Part model, mm, in its own coordinate system. Face numbers are marked on the shaded views. A direction names the side the tool comes from. Round coordinates to 2 decimals unless told otherwise and drop trailing zeros. Loops run counter-clockwise (first coordinate to the right, second up) from the corner with the lowest first, then second, coordinate; pieces in that order, holes last.
1) Drop flat-ended pins along their axis: P1, Ø3, axis at y = 2.5, z = -12, coming from the +X side; P2, Ø6, axis at x = -5.5, z = -9, coming from the -Y side; P3, Ø4, axis at x = -2, y = 13, coming from the -Z side. Give the stop position or say it passes through.
2) 3-axis set-ups, long thin cutter, end or side, ignore diameter. For the marked faces 4, 5 and 6: which of +Z, -Z, +X, -X, +Y, -Y reach the whole face in a straight line?
3) Band-saw the part on B-B, the plane z = 0. Write the cut outline in (x, y), then the cut area to 3 significant figures.
4) Mould opens along X. For the marked faces 1, 2 and 3 say: +X half, -X half, draft (parallel to the pull), parting line (faces both ways), or undercut.
5) Band-saw the part on C-C, the plane y = 7.75. Write the cut outline in (x, z), then the cut area to 3 significant figures.
6) Probe line 1 (Y direction, x = 0, z = 9.5); line 2 (X direction, y = 6.25, z = 0); line 3 (X direction, y = 0.5, z = 0). List the from-to ranges inside material, lowest first.
7) Band-saw the part on D-D, the plane y = 4. Write the cut outline in (x, z).
8) Band-saw the part on A-A, the plane x = 0. Write the cut outline in (y, z), then the cut area to 3 significant figures.
from build123d import *

# Parameters (mm, degrees)
SKETCH1_R             = 7.5
BASE_CYLINDER_DEPTH   = 15.4
LED_HOLDER_DEPTH      = 7.5
LED_HOLDER_DEPTH_BACK = 22.5
F_3DSKETCH2_R         = 3.5
SKETCH2_R             = 6.05
CUT_EXTRUDE1_DEPTH    = 14.2
CUT_EXTRUDE2_REACH    = 24.769
SKETCH3_R             = 1.75
SKETCH4_R             = 2.5
CUT_EXTRUDE3_DEPTH    = 35.545766898


with BuildPart() as part:
    # Sketch1 → base-cylinder (new body)
    with BuildSketch(Plane(origin=(0, 0, 0), x_dir=(1, 0, 0), z_dir=(0, 1, 0))):
        with Locations(Location((0, 0, 0), (0, 0, 90))):
            Circle(SKETCH1_R)
    extrude(amount=BASE_CYLINDER_DEPTH)

    # 3DSketch2 → led-holder (add, two sides: drawn at the far end of the back side and taken through both)
    with BuildSketch(Plane(origin=(-3.5, 4.7, 7.5), x_dir=(0.894427190999916, -0.44721359549995804, 0), z_dir=(0, 0, 1)).offset(-LED_HOLDER_DEPTH_BACK)):
        with Locations((3.130495168, 1.565247584)):
            Circle(F_3DSKETCH2_R)
        Polygon((0, 0), (6.260990337, 3.130495168), (7.826237921, 0), (1.565247584, -3.130495168), align=None)
    extrude(amount=LED_HOLDER_DEPTH + LED_HOLDER_DEPTH_BACK)

    # Sketch2 → Cut-Extrude1 (cut)
    with BuildSketch(Plane(origin=(0, 15.4, 0), x_dir=(1, 0, 0), z_dir=(0, 1, 0))):
        with Locations(Location((0, 0, 0), (0, 0, 270))):
            Circle(SKETCH2_R)
    extrude(amount=-CUT_EXTRUDE1_DEPTH, mode=Mode.SUBTRACT)

    # Sketch3 → Cut-Extrude2 (cut, up to next)
    with BuildSketch(Plane.XZ, mode=Mode.PRIVATE) as cut_extrude2_sk1:
        with Locations(Location((0, 0, 0), (0, 0, 270))):
            Circle(SKETCH3_R)
    cut_extrude2_tool1 = extrude(cut_extrude2_sk1.sketch, amount=-CUT_EXTRUDE2_REACH, mode=Mode.PRIVATE) & part.part
    add(cut_extrude2_tool1.solids().sort_by_distance((0, 0, 0))[0], mode=Mode.SUBTRACT)

    # Sketch4 → Cut-Extrude3 (cut, through all)
    with BuildSketch(Plane(origin=(0, 0, -15), x_dir=(-1, 0, 0), z_dir=(0, 0, -1))):
        with Locations((0, 4.7)):
            Circle(SKETCH4_R)
    extrude(amount=-CUT_EXTRUDE3_DEPTH, mode=Mode.SUBTRACT)


solid = part.part
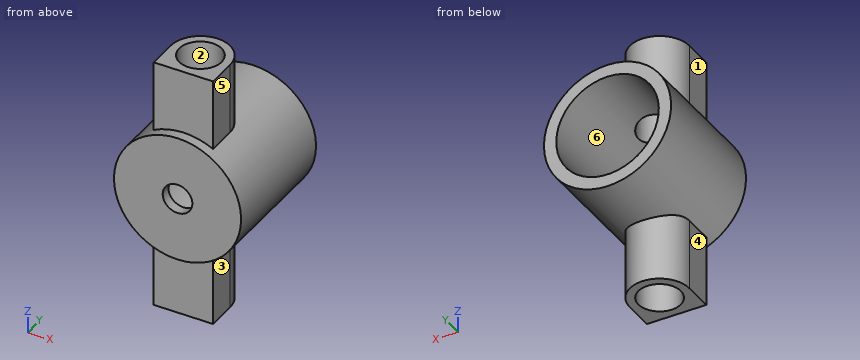
Reported:
1. P1: stops at x = 3.5
1. P2: stops at y = 1.2
1. P3: stops at z = -7.5
2. face 4: -Z, -X, +Y, -Y
2. face 5: +Z, +X, +Y, -Y
2. face 6: +Y
3. outline: (-7.5, 0) - (-1.75, 0) - (-1.75, 1.2) - (-6.05, 1.2) - (-6.05, 15.4) - (-7.5, 15.4) - close; (1.75, 0) - (7.5, 0) - (7.5, 15.4) - (6.05, 15.4) - (6.05, 1.2) - (1.75, 1.2) - close
3. area: 55.0 mm2
4. face 1: -X half
4. face 2: undercut
4. face 3: +X half
5. outline: (-1.72, -15) - (1.72, -15) - (1.72, -7.3) arc R7.5 ccw to (1.72, 7.3) - (1.72, 15) - (-1.72, 15) - (-1.72, 7.3) arc R7.5 ccw to (-1.72, -7.3) - close; hole circle Ø12.1 at (0, 0)
5. area: 114 mm2
6. line 1: y = 1.2 to 2.2, 7.2 to 8.2
6. line 2: x = -7.5 to -6.05, 6.05 to 7.5
6. line 3: x = -7.5 to -1.75, 1.75 to 7.5
7. outline: (-3.5, -15) - (-2.4, -15) - (-2.4, -5.55) arc R6.05 cw to (-2.4, 5.55) - (-2.4, 15) - (-3.5, 15) - (-3.5, 6.63) arc R7.5 ccw to (-3.5, -6.63) - close; (2.4, -15) - (3.5, -15) - (3.5, -6.63) arc R7.5 ccw to (3.5, 6.63) - (3.5, 15) - (2.4, 15) - (2.4, 5.55) arc R6.05 cw to (2.4, -5.55) - close
8. outline: (0, -7.5) - (1.2, -7.5) - (1.2, -15) - (2.2, -15) - (2.2, -6.05) - (1.2, -6.05) - (1.2, -1.75) - (0, -1.75) - close; (0, 1.75) - (1.2, 1.75) - (1.2, 6.05) - (2.2, 6.05) - (2.2, 15) - (1.2, 15) - (1.2, 7.5) - (0, 7.5) - close; (7.2, -15) - (8.2, -15) - (8.2, -7.5) - (15.4, -7.5) - (15.4, -6.05) - (7.2, -6.05) - close; (7.2, 6.05) - (15.4, 6.05) - (15.4, 7.5) - (8.2, 7.5) - (8.2, 15) - (7.2, 15) - close
8. area: 70.5 mm2
